Autodesk Inventor part; units mm, degrees
ref_plane "YZ Plane" through (0, 0, 0) normal (1, 0, 0) x (0, 1, 0)
ref_plane "XZ Plane" through (0, 0, 0) normal (0, 1, 0) x (-1, 0, 0)
ref_plane "XY Plane" through (0, 0, 0) normal (0, 0, 1) x (1, 0, 0)
sketch "Sketch1" plane through (0, 0, 0) normal (1, 0, 0) x (0, 1, 0)
  line L0 (-13.6199, 37.7174) -> (-13.6199, 37.7021)
  line L1 (-13.6199, 37.7021) -> (-13.6199, 37.664)
  line L2 (-13.6199, 37.664) -> (-13.6199, 37.6513)
  line L3 (-13.6199, 37.6513) -> (-13.6226, 37.0747)
  line L4 (-13.6226, 37.0747) -> (-13.1538, 35.3425)
  line L5 (-13.1538, 35.3425) -> (-11.8683, 33.4806)
  line L6 (-11.8683, 33.4806) -> (-9.9635, 32.2767)
  line L7 (-9.9635, 32.2767) -> (-8.2163, 31.8957)
  line L8 (-8.2163, 31.8957) -> (-7.643, 31.9312)
  line L9 (-7.643, 31.9312) -> (-6.3367, 32.0125)
  line L10 (-6.3367, 32.0125) -> (-2.4121, 32.2564)
  line L11 (-2.4121, 32.2564) -> (3.3634, 32.6094)
  line L12 (3.3634, 32.6094) -> (9.1619, 32.9625)
  line L13 (9.1619, 32.9625) -> (13.1363, 33.1987)
  line L14 (13.1363, 33.1987) -> (14.4621, 33.2774)
  line L15 (14.4621, 33.2774) -> (15.4583, 33.3359)
  line L16 (15.4583, 33.3359) -> (18.4512, 33.5111)
  line L17 (18.4512, 33.5111) -> (22.3554, 33.7423)
  line L18 (22.3554, 33.7423) -> (26.0527, 33.9607)
  line L19 (26.0527, 33.9607) -> (29.4232, 34.1614)
  line L20 (29.4232, 34.1614) -> (32.3475, 34.3417)
  line L21 (32.3475, 34.3417) -> (34.7054, 34.489)
  line L22 (34.7054, 34.489) -> (36.3755, 34.6008)
  line L23 (36.3755, 34.6008) -> (37.0247, 34.649)
  line L24 (37.0247, 34.649) -> (37.2396, 34.6719)
  line L25 (37.2396, 34.6719) -> (38.0554, 34.7633)
  line L26 (38.0554, 34.7633) -> (40.4847, 35.2307)
  line L27 (40.4847, 35.2307) -> (42.8482, 36.0029)
  line L28 (42.8482, 36.0029) -> (44.2921, 36.8715)
  line L29 (44.2921, 36.8715) -> (44.7829, 37.5142)
  line L30 (44.7829, 37.5142) -> (44.7829, 37.725)
  line L31 (44.7829, 37.725) -> (44.7829, 37.9383)
  line L32 (44.7829, 37.9383) -> (44.2921, 38.5708)
  line L33 (44.2921, 38.5708) -> (42.8482, 39.4395)
  line L34 (42.8482, 39.4395) -> (40.4847, 40.2091)
  line L35 (40.4847, 40.2091) -> (38.0554, 40.6739)
  line L36 (38.0554, 40.6739) -> (37.2396, 40.7654)
  line L37 (37.2396, 40.7654) -> (37.0247, 40.7908)
  line L38 (37.0247, 40.7908) -> (36.3755, 40.8365)
  line L39 (36.3755, 40.8365) -> (34.7042, 40.9508)
  line L40 (34.7042, 40.9508) -> (32.3448, 41.0981)
  line L41 (32.3448, 41.0981) -> (29.4177, 41.2784)
  line L42 (29.4177, 41.2784) -> (26.0445, 41.4791)
  line L43 (26.0445, 41.4791) -> (22.343, 41.6975)
  line L44 (22.343, 41.6975) -> (18.436, 41.9287)
  line L45 (18.436, 41.9287) -> (15.4418, 42.1039)
  line L46 (15.4418, 42.1039) -> (14.4441, 42.1624)
  line L47 (14.4441, 42.1624) -> (13.1197, 42.2386)
  line L48 (13.1197, 42.2386) -> (9.1482, 42.4773)
  line L49 (9.1482, 42.4773) -> (3.3547, 42.8278)
  line L50 (3.3547, 42.8278) -> (-2.4149, 43.1834)
  line L51 (-2.4149, 43.1834) -> (-6.3367, 43.4273)
  line L52 (-6.3367, 43.4273) -> (-7.643, 43.5086)
  line L53 (-7.643, 43.5086) -> (-8.2163, 43.5441)
  line L54 (-8.2163, 43.5441) -> (-9.9635, 43.1631)
  line L55 (-9.9635, 43.1631) -> (-11.8683, 41.9566)
  line L56 (-11.8683, 41.9566) -> (-13.1538, 40.0973)
  line L57 (-13.1538, 40.0973) -> (-13.6226, 38.3625)
  line L58 (-13.6226, 38.3625) -> (-13.6199, 37.7859)
  line L59 (-13.6199, 37.7859) -> (-13.6199, 37.7682)
  line L60 (-13.6199, 37.7682) -> (-13.6199, 37.7326)
  line L61 (-13.6199, 37.7326) -> (-13.6199, 37.7174)
  line L62 (-14.0082, 28.1898) -> (-14.295, 28.6115)
  line L63 (-14.295, 28.6115) -> (-14.4575, 28.8502)
  line L64 (-14.4575, 28.8502) -> (-14.5541, 28.9925)
  line L65 (-14.5541, 28.9925) -> (-15.0049, 29.5817)
extrude "Extrusion27" add sketch "Sketch1" along normal blind 0.25
sketch "Sketch7" plane through (0, 0, 0) normal (-1, 0, 0) x (0, 0, 1)
  circle A0 centre (37.7743, -8.0049) radius 5.5
  circle A1 centre (37.7743, -8.0049) radius 0.5
  point P0 (0, 0)
  dimension "d91" = 11
  dimension "d92" = 1
extrude "Extrusion30" [suppressed]
properties part number "Sticker6"
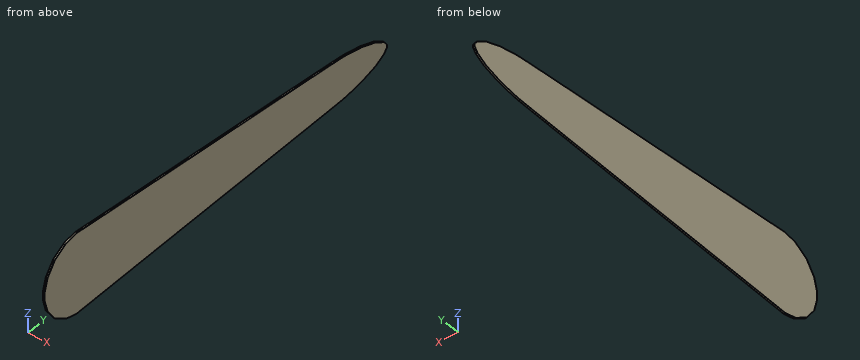
Design review of the part built by this model. Coordinates are the model's own, in mm. Give positions to 0.01 mm unless a question says otherwise; leave off trailing zeros. Order: outer loops, then holes, each group sorted by start corner. A loop starts at its lowest first (then second) coordinate and runs counter-clockwise, first axis right, second up.
1. Add section A-A, the plane y = 7. State the section outline as (x, z) points, then the cut area to 3 significant figures.
Solution:
outline: (0, 32.83) - (0.25, 32.83) - (0.25, 42.61) - (0, 42.61) - close
area: 2.44 mm2
2. Add section B-B, the plane y = 41.5. State the section outline as (x, z) points, then the cut area to 3 significant figures.
Solution:
outline: (0, 35.56) - (0.25, 35.56) - (0.25, 39.88) - (0, 39.88) - close
area: 1.08 mm2
3. To check wall thickness, follow L1, parallel to Z at x = 0.2, y = 10; L2, parallel to Z at x = 0.15, y = 12; L3, parallel to Y at x = 0.1, z = 37.25. State the ranges of each line that lie inside material, in increasing order.
Solution:
L1: z = 33.01 to 42.43
L2: z = 33.13 to 42.31
L3: y = -13.62 to 44.58
4. For pin 1 Ø6 at (y, z) = (24.5, 42) entering from -X, flat-tipped, find the tip position at first contact; note if it passes through.
Solution:
pin 1: stops at x = 0
